Could you check a few things on this model? Use its own coordinates, in mm. A direction names the side the tool comes from. Round coordinates to 2 decimals unless told otherwise and drop trailing zeros. Write each loop counter-clockwise with the first axis right and the second up, starting at its lowest first coordinate (ties: lowest second). Pieces come first, ordered by that corner, then holes. Notation, with made-up numbers: (71.25, 72) -> (84.25, 72) arc R6 cw to (84.25, 81) -> close; hole circle Ø9 at (-14.5, 12). An arc over 180 degrees is marked (long way). Answer in a Markdown table with one row per item.
from build123d import *

# Parameters (mm, degrees)
SKETCH1_W           = 2.5
SKETCH1_H           = 5
SKETCH1_W_2         = 12.691848092
SKETCH1_H_2         = 2
BOSS_EXTRUDE1_DEPTH = 10
BOSS_EXTRUDE2_DEPTH = 5
LPATTERN1_COUNT     = 5
LPATTERN1_PITCH     = 2


with BuildPart() as part:
    # Sketch1 → Boss-Extrude1 (new body)
    # profile 1 of 3: a face of its own
    with BuildSketch(Plane.XY):
        Polygon((49.805812864, -41.856488388), (49.805812864, -39.856488388), (47.805812864, -39.856488388), (47.805812864, -36.356488388), (41.305812864, -36.356488388), (41.305812864, -45.356488388), (47.805812864, -45.356488388), (47.805812864, -41.856488388), align=None)
        with Locations((44.555812864, -40.856488388)):
            Rectangle(SKETCH1_W, SKETCH1_H, mode=Mode.SUBTRACT)
    # profile 2 of 3: a face of its own
    with BuildSketch(Plane.XY):
        Polygon((66.497660956, -33.227883866), (49.805812864, -29.527390234), (49.805812864, -39.856488388), (49.805812864, -41.856488388), (49.805812864, -52.138716904), (66.497660956, -48.438223273), align=None)
        Polygon((51.805812864, -41.856488388), (51.805812864, -39.856488388), (51.805812864, -32.019338588), (64.497660956, -34.833053569), (64.497660956, -39.856488388), (64.497660956, -41.856488388), (64.497660956, -46.833053569), (51.805812864, -49.64676855), align=None, mode=Mode.SUBTRACT)
    # profile 3 of 3: a face of its own
    with BuildSketch(Plane.XY):
        with Locations((58.15173691, -40.856488388)):
            Rectangle(SKETCH1_W_2, SKETCH1_H_2)
    extrude(amount=BOSS_EXTRUDE1_DEPTH)

    # Sketch2 → Boss-Extrude2 (add)
    with BuildSketch(Plane.XZ.offset(38.356488388)):
        with BuildLine():
            Line((43.305812864, 8.8), (43.305812864, 10))
            ThreePointArc((43.305812864, 10), (43.905812864, 9.4), (43.305812864, 8.8))
        make_face()
    boss_extrude2 = extrude(amount=BOSS_EXTRUDE2_DEPTH)

    # LPattern1: Boss-Extrude2 ×5
    with Locations(*[(0, 0, -i * LPATTERN1_PITCH) for i in range(1, LPATTERN1_COUNT)]):
        add(boss_extrude2)


solid = part.part
1) Imagine slicing it at A-A, the plane y = -35.5. Please give me the cut outline in (x, z).
Findings:
| item | result |
|---|---|
| outline | (49.81, 0) -> (51.81, 0) -> (51.81, 10) -> (49.81, 10) -> close; (64.5, 0) -> (66.5, 0) -> (66.5, 10) -> (64.5, 10) -> close |
2) Thinking about a two-plate mould opening in Y: for faces 6 (the face through (49, -41.856, 5)), 7 (the face through (49.806, -35, 5)), 8 (the face through (58.24, -48.22, 4.93)), which applies, +Y half, -Y half, draft (parallel to the pull), parting line (faces both ways), or undercut?
Findings:
| item | result |
|---|---|
| face 6 | -Y half |
| face 7 | draft |
| face 8 | undercut |
3) For pin 1 (2 mm diameter, centred on x = 48.5, z = 5, fed in from -Y); pin 2 (3 mm diameter, centred on y = -34.5, z = 5.5, fed in from -X); pin 3 (2 mm diameter, centred on x = 48.5, z = 4.5, fed in from +Y), each with a flat end and sliding along its axis, tell me the tip position at first contact or that it passes through.
Findings:
| item | result |
|---|---|
| pin 1 | stops at y = -45.36 |
| pin 2 | stops at x = 49.81 |
| pin 3 | stops at y = -36.36 |
4) For faces 1 (the face through (43.306, -40.9, 8.4)), 2 (the face through (57, -41, 10)), 3 (the face through (41.306, -41, 5)), 4 (the face through (49.806, -47, 5)), 5 (the face through (64.498, -37, 5)), which set-ups out of +Z, -Z, +X, -X, +Y, -Y let a thin tool reach every point of the face, with its end or its side?
Findings:
| item | result |
|---|---|
| face 1 | none |
| face 2 | +Z, +X, -X, +Y, -Y |
| face 3 | +Z, -Z, -X, +Y, -Y |
| face 4 | +Z, -Z, -Y |
| face 5 | +Z, -Z |
5) Imagine slicing it at C-C, the plane y = -43. Please give me the cut outline in (x, z), plus the area to 3 significant figures.
Findings:
| item | result |
|---|---|
| outline | (41.31, 0) -> (43.31, 0) -> (43.31, 0.8) arc R0.6 ccw to (43.31, 2) -> (43.31, 2.8) arc R0.6 ccw to (43.31, 4) -> (43.31, 4.8) arc R0.6 ccw to (43.31, 6) -> (43.31, 6.8) arc R0.6 ccw to (43.31, 8) -> (43.31, 8.8) arc R0.6 ccw to (43.31, 10) -> (41.31, 10) -> close; (45.81, 0) -> (47.81, 0) -> (47.81, 10) -> (45.81, 10) -> close; (49.81, 0) -> (51.81, 0) -> (51.81, 10) -> (49.81, 10) -> close; (64.5, 0) -> (66.5, 0) -> (66.5, 10) -> (64.5, 10) -> close |
| area | 82.8 mm^2 |
6) Please list where these lines run through material, in increasing order: line 1 (X direction, y = -38.75, z = 8.75); line 2 (X direction, y = -36, z = 7); line 3 (X direction, y = -40, z = 4.75).
Findings:
| item | result |
|---|---|
| line 1 | x = 41.31 to 43.31, 45.81 to 47.81, 49.81 to 51.81, 64.5 to 66.5 |
| line 2 | x = 49.81 to 51.81, 64.5 to 66.5 |
| line 3 | x = 41.31 to 43.31, 45.81 to 66.5 |
7) Imagine slicing it at B-B, the plane z = 1.4. Please give me the cut outline in (x, y), plus the area to 3 significant figures.
Findings:
| item | result |
|---|---|
| outline | (41.31, -45.36) -> (47.81, -45.36) -> (47.81, -41.86) -> (49.81, -41.86) -> (49.81, -52.14) -> (66.5, -48.44) -> (66.5, -33.23) -> (49.81, -29.53) -> (49.81, -39.86) -> (47.81, -39.86) -> (47.81, -36.36) -> (41.31, -36.36) -> close; hole (43.91, -43.36) -> (45.81, -43.36) -> (45.81, -38.36) -> (43.91, -38.36) -> close; hole (51.81, -49.65) -> (64.5, -46.83) -> (64.5, -41.86) -> (51.81, -41.86) -> close; hole (51.81, -39.86) -> (64.5, -39.86) -> (64.5, -34.83) -> (51.81, -32.02) -> close |
| area | 206 mm^2 |
8) Imagine slicing it at D-D, the plane x = 58. Please give me the cut outline in (y, z), plus the area to 3 significant figures.
Findings:
| item | result |
|---|---|
| outline | (-50.32, 0) -> (-48.27, 0) -> (-48.27, 10) -> (-50.32, 10) -> close; (-41.86, 0) -> (-39.86, 0) -> (-39.86, 10) -> (-41.86, 10) -> close; (-33.39, 0) -> (-31.34, 0) -> (-31.34, 10) -> (-33.39, 10) -> close |
| area | 61.0 mm^2 |
